Source: CAD feature listing. Evaluate the final solid. Frame: model axes, mm. Face numbers are marked on the shaded views. A direction names the side the tool comes from. Round coordinates to 2 decimals unless told otherwise and drop trailing zeros. Loops run counter-clockwise (first coordinate to the right, second up) from the corner with the lowest first, then second, coordinate; pieces in that order, holes last. Notation, with made-up numbers: M 73.5,-9.5 L 86.5,-9.5 A23 ccw 86.5,11.5 Z; hole C 69,-6 d9. An arc over 180 degrees is marked long. One line per item, written item: value.
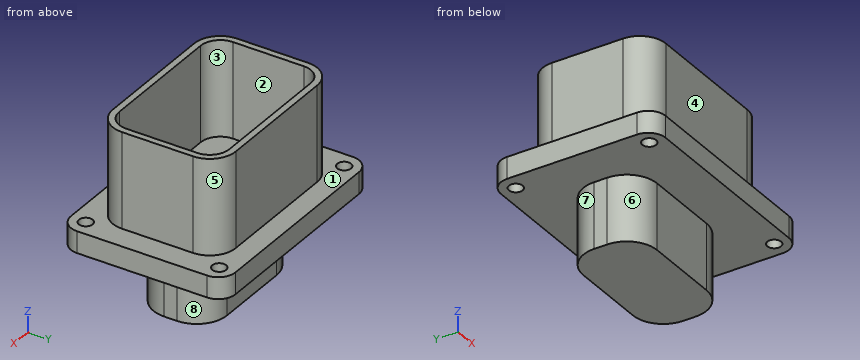
from build123d import *

# Parameters (mm, degrees)
SKETCH1_W           = 52
SKETCH1_H           = 38
SKETCH1_R           = 1.6
BOSS_EXTRUDE1_DEPTH = 5
SKETCH5_W           = 31.6
SKETCH5_H           = 17
BOSS_EXTRUDE2_DEPTH = 15.2
BOSS_EXTRUDE3_DEPTH = 22
FILLET1_R           = 4
FILLET2_R           = 7


with BuildPart() as part:
    # Sketch1 → Boss-Extrude1 (new body)
    with BuildSketch(Plane.XY):
        with Locations((26, 19)):
            Rectangle(SKETCH1_W, SKETCH1_H)
        with Locations((3.75, 34.4)):
            Circle(SKETCH1_R, mode=Mode.SUBTRACT)
        with Locations((48.25, 34.4)):
            Circle(SKETCH1_R, mode=Mode.SUBTRACT)
        with Locations((48.25, 3.6)):
            Circle(SKETCH1_R, mode=Mode.SUBTRACT)
        with Locations((3.75, 3.6)):
            Circle(SKETCH1_R, mode=Mode.SUBTRACT)
    extrude(amount=BOSS_EXTRUDE1_DEPTH)

    # Sketch5 → Boss-Extrude2 (add)
    with BuildSketch(Plane(origin=(0, 0, 0), x_dir=(-1, 0, 0), z_dir=(0, 0, -1))):
        with Locations((-26, 19)):
            Rectangle(SKETCH5_W, SKETCH5_H)
    extrude(amount=BOSS_EXTRUDE2_DEPTH)

    # Sketch7 → Boss-Extrude3 (add)
    with BuildSketch(Plane.XY.offset(5)):
        with BuildLine():
            Line((11.5, 33.188764045), (40.5, 33.188764045))
            ThreePointArc((40.5, 33.188764045), (44.742640687, 31.431404732), (46.5, 27.188764045))
            Line((46.5, 27.188764045), (46.5, 10.811235955))
            ThreePointArc((46.5, 10.811235955), (44.742640687, 6.568595268), (40.5, 4.811235955))
            Line((40.5, 4.811235955), (11.5, 4.811235955))
            ThreePointArc((11.5, 4.811235955), (7.257359313, 6.568595268), (5.5, 10.811235955))
            Line((5.5, 10.811235955), (5.5, 27.188764045))
            ThreePointArc((5.5, 27.188764045), (7.257359313, 31.431404732), (11.5, 33.188764045))
        make_face()
        with BuildLine():
            Line((11.5, 31.688764045), (40.5, 31.688764045))
            ThreePointArc((40.5, 31.688764045), (43.681980515, 30.37074456), (45, 27.188764045))
            Line((45, 27.188764045), (45, 10.811235955))
            ThreePointArc((45, 10.811235955), (43.681980515, 7.62925544), (40.5, 6.311235955))
            Line((40.5, 6.311235955), (11.5, 6.311235955))
            ThreePointArc((11.5, 6.311235955), (8.318019485, 7.62925544), (7, 10.811235955))
            Line((7, 10.811235955), (7, 27.188764045))
            ThreePointArc((7, 27.188764045), (8.318019485, 30.37074456), (11.5, 31.688764045))
        make_face(mode=Mode.SUBTRACT)
    extrude(amount=BOSS_EXTRUDE3_DEPTH)

    # Fillet1
    fillet1_edges = [part.edges().sort_by_distance(p)[0] for p in [
        (0, 0, 2.5),
        (0, 38, 2.5),
        (52, 38, 2.5),
        (52, 0, 2.5),
    ]]
    fillet(fillet1_edges, radius=FILLET1_R)

    # Fillet2
    fillet2_edges = [part.edges().sort_by_distance(p)[0] for p in [
        (41.8, 27.5, -7.6),
        (41.8, 10.5, -7.6),
        (10.2, 10.5, -7.6),
        (10.2, 27.5, -7.6),
    ]]
    fillet(fillet2_edges, radius=FILLET2_R)


solid = part.part
1. Pin query (flat end, axial travel): pin 1 (0.9 mm diameter, centred on y = 18.5, z = -11, fed in from -X); pin 2 (8 mm diameter, centred on y = 7.5, z = 12.5, fed in from +X); pin 3 (3 mm diameter, centred on y = 11, z = 17, fed in from -X). Return the tip coordinate at first contact, or that it passes through.
Report:
pin 1: stops at x = 10.2
pin 2: stops at x = 46.5
pin 3: stops at x = 5.5
2. Section query B-B (x = 32). Return the cut outline in (y, z).
Report:
outline: M 0,0 L 10.5,0 L 10.5,-15.2 L 27.5,-15.2 L 27.5,0 L 38,0 L 38,5 L 33.19,5 L 33.19,27 L 31.69,27 L 31.69,5 L 6.31,5 L 6.31,27 L 4.81,27 L 4.81,5 L 0,5 Z
3. Reachability of the marked faces 5, 6, 7 and 8 from +Z, -Z, +X, -X, +Y, -Y: full face, straight path, thin tool, end or side. Return the list, or none.
Report:
face 5: +Z, +X, +Y
face 6: -Z, -X, -Y
face 7: -Z, -X, +Y
face 8: -Z, +X, +Y
4. Section query A-A (z = 1). Return the cut outline in (x, y), and give its area (3 significant figures).
Report:
outline: M 0,4 A4 ccw 4,0 L 48,0 A4 ccw 52,4 L 52,34 A4 ccw 48,38 L 4,38 A4 ccw 0,34 Z; hole C 3.75,3.6 d3.2; hole C 3.75,34.4 d3.2; hole C 48.25,3.6 d3.2; hole C 48.25,34.4 d3.2
area: 1,930 mm2
5. Section query D-D (z = -9). Return the cut outline in (x, y), and give its area (3 significant figures).
Report:
outline: M 10.2,17.5 A7 ccw 17.2,10.5 L 34.8,10.5 A7 ccw 41.8,17.5 L 41.8,20.5 A7 ccw 34.8,27.5 L 17.2,27.5 A7 ccw 10.2,20.5 Z
area: 495 mm2
6. Ray query, line 1 (Y direction, x = 15, z = 11); line 2 (Y direction, x = 48.25, z = 2.4); line 3 (X direction, y = 23, z = 8). Return the intervals inside material, ascending. Write a range as [from, to].
Report:
line 1: y = [4.81, 6.31], [31.69, 33.19]
line 2: y = [0.01, 2], [5.2, 32.8], [36, 37.99]
line 3: x = [5.5, 7], [45, 46.5]
7. Section query C-C (z = 20). Return the cut outline in (x, y), and give its area (3 significant figures).
Report:
outline: M 5.5,10.81 A6 ccw 11.5,4.81 L 40.5,4.81 A6 ccw 46.5,10.81 L 46.5,27.19 A6 ccw 40.5,33.19 L 11.5,33.19 A6 ccw 5.5,27.19 Z; hole M 7,10.81 A4.5 ccw 11.5,6.31 L 40.5,6.31 A4.5 ccw 45,10.81 L 45,27.19 A4.5 ccw 40.5,31.69 L 11.5,31.69 A4.5 ccw 7,27.19 Z
area: 186 mm2
8. Pull-direction query (Y, two-part tool) for the marked faces 1, 2, 3 and 4; classes: released by +Y, released by -Y, zero draft, split by the parting line, or undercut.
Report:
face 1: zero draft
face 2: undercut
face 3: undercut
face 4: released by -Y
